For this review, use the dimensioned drawing (mm, ordinates from the lowest corner) and the shaded views. A direction names the side the tool comes from. Round coordinates to 2 decimals unless told otherwise and drop trailing zeros. Loops run counter-clockwise (first coordinate to the right, second up) from the corner with the lowest first, then second, coordinate; pieces in that order, holes last. Notation, with made-up numbers: (-33.5, 9.25) -> (13.5, 9.25) arc R19 cw to (13.5, 30.25) -> close; hole circle Ø1 at (78.25, -32). An arc over 180 degrees is marked (long way). Write each question's results on one line, items separated by ' | '. Start each with the question number.
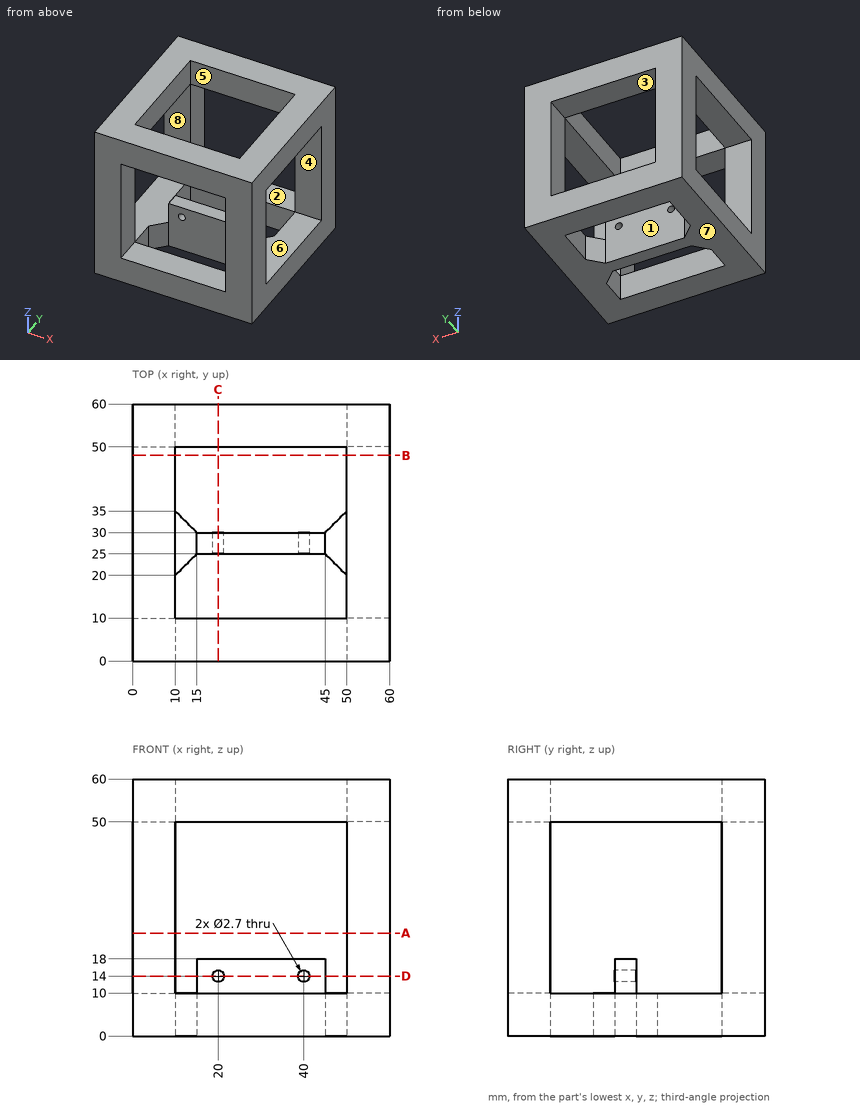
1) Take a section at D-D (z = 14). Write out the cut boundary in (x, y).
2) Take a section at C-C (x = 20). Write out the cut boundary in (y, z), plus the area to 4 significant figures.
3) For the marked faces 1, 2, 3 and 4, list the 3-axis set-ups (+Z, -Z, +X, -X, +Y, -Y) from which the entire face can be reached by the end or side of a thin tool; tool diameter is ignored.
4) The part is to be moulded in two halves that separate along Z. For the marked faces 5, 6, 7 and 8, say which applies: +Z half, -Z half, draft (parallel to the pull), parting line (faces both ways), or undercut.
5) To check wall thickness, follow line 1 (X direction, y = 27.6, z = 14); line 2 (Y direction, x = 35, z = 8.5); line 3 (Y direction, x = 39.5, z = 53). State the ranges of each line that lie inside material, in increasing order. Write a range as from..to.
6) Take a section at A-A (z = 24). Write out the cut boundary in (x, y), plus the area to 3 significant figures.
7) Insertion check: pin 1 (1 mm diameter, centred on x = 47.5, z = 48.5, fed in from -Y); pin 2 (3 mm diameter, centred on x = 40, z = 14, fed in from -Y); pin 3 (4 mm diameter, centred on y = 27.5, z = 13, fed in from +X). Each pin has a flat end and moves straight along its axis. Give the tip position at first contact, or say it passes through.
Geometry check:
1) outline: (0, 0) -> (10, 0) -> (10, 10) -> (0, 10) -> close; (0, 50) -> (10, 50) -> (10, 60) -> (0, 60) -> close; (15, 25) -> (18.65, 25) -> (18.65, 30) -> (15, 30) -> close; (21.35, 25) -> (38.65, 25) -> (38.65, 30) -> (21.35, 30) -> close; (41.35, 25) -> (45, 25) -> (45, 30) -> (41.35, 30) -> close; (50, 0) -> (60, 0) -> (60, 10) -> (50, 10) -> close; (50, 50) -> (60, 50) -> (60, 60) -> (50, 60) -> close
2) outline: (0, 0) -> (10, 0) -> (10, 10) -> (0, 10) -> close; (0, 50) -> (10, 50) -> (10, 60) -> (0, 60) -> close; (25, 0) -> (30, 0) -> (30, 12.65) -> (25, 12.65) -> close; (25, 15.35) -> (30, 15.35) -> (30, 18) -> (25, 18) -> close; (50, 0) -> (60, 0) -> (60, 10) -> (50, 10) -> close; (50, 50) -> (60, 50) -> (60, 60) -> (50, 60) -> close | area: 476.5 mm^2
3) face 1: +Z, -Z | face 2: +Y | face 3: +Y, -Y | face 4: +X, -X
4) face 5: draft | face 6: undercut | face 7: -Z half | face 8: undercut
5) line 1: x = 15..18.65, 21.35..38.65, 41.35..45 | line 2: y = 0..10, 25..30, 50..60 | line 3: y = 0..10, 50..60
6) outline: (0, 0) -> (10, 0) -> (10, 10) -> (0, 10) -> close; (0, 50) -> (10, 50) -> (10, 60) -> (0, 60) -> close; (50, 0) -> (60, 0) -> (60, 10) -> (50, 10) -> close; (50, 50) -> (60, 50) -> (60, 60) -> (50, 60) -> close | area: 400 mm^2
7) pin 1: passes through | pin 2: stops at y = 25 | pin 3: stops at x = 45
